Part model, mm, in its own coordinate system. A direction names the side the tool comes from. Coordinates: 2 decimals unless noted, no trailing zeros. Loops run counter-clockwise (first coordinate to the right, second up) from the corner with the lowest first, then second, coordinate; pieces in that order, holes last. Notation, with made-up numbers: M 86,5 L 105,5 A9 ccw 105,14 Z; hole C -5.5,50 d11. An arc over 180 degrees is marked long. Use a Markdown table: item, result. Add a question column.
1) Pull direction Z, two halves, no side cores. Call faces 6 (the cylindrical face through (-0.147, 1.61, 32.217)), 7 (the cylindrical face through (-30.235, 1.565, 23.183)), 8 (the flat face through (16.4, 3.175, 16.4)): released by +Z, released by -Z, zero draft, split by the parting line, or undercut.
2) Band-saw the part on D-D (z = -30). List the corners of the cut face in (x, y) (3 decimals), plus the area to 3 significant figures.
3) Pin check, flat tips, straight feed: pin 1 Ø10 at (x, y) = (-6.5, 10.5) entering from -Z; pin 2 Ø1.8 at (x, y) = (-17.78, 5.715) entering from -Z; pin 3 Ø2 at (y, z) = (5.715, -17.78) entering from +X. Stop position of each tip, or through.
4) Band-saw the part on C-C (y = 11.25). List the corners of the cut face in (x, z), plus the area to 3 significant figures.
5) Wall check: probe 1 along Y at (x, z) = (14, -28.5) (3 decimals); probe 2 along Z at (x, y) = (-16.5, 3.5); probe 3 along Z at (x, y) = (-2.5, 1.5). Give the ranges that are in metal, low to high. Write a range as from..to.
6) Band-saw the part on A-A (x = 0). List the corners of the cut face in (y, z) (3 decimals).
7) Tool access for faces 1 (the flat face through (0, 8.255, 0)), 2 (the cylindrical face through (21.804, 6.619, -6.867)), 3 (the cylindrical face through (18.9, 5.57, -10.56)), 4 (the cylindrical face through (-18.9, 5.57, 10.56)), 5 (the cylindrical face through (10.56, 5.57, 18.9)): list every direction of +Z, -Z, +X, -X, +Y, -Y with a clear straight run to the whole face (end or side of a thin tool).
8) Band-saw the part on B-B (y = 2). State how many separate pieces and enclosed holes the cut face has, plus the area to 3 significant figures.
from build123d import *

# Parameters (mm, degrees)
SKETCH2_R                 = 38.1
BOSS_EXTRUDE1_DEPTH       = 3.175
TAP_DRILL_FOR_4_40_TAP1_D = 2.2606
CIRPATTERN1_COUNT         = 8
SKETCH7_R                 = 22.86
BOSS_EXTRUDE2_DEPTH       = 6.985
SKETCH8_R                 = 19.05
CUT_EXTRUDE1_DEPTH        = 8.255
SKETCH12_W                = 1.1303
SKETCH12_H                = 38.1
CIRPATTERN2_COUNT         = 4
SKETCH14_R                = 5.08
SKETCH13_R                = 22.86


with BuildPart() as part:
    # Sketch2 → Boss-Extrude1 (new body)
    with BuildSketch(Plane(origin=(0, 0, 0), x_dir=(1, 0, 0), z_dir=(0, 1, 0))):
        Circle(SKETCH2_R)
    extrude(amount=BOSS_EXTRUDE1_DEPTH)

    # Tap Drill for #4-40 Tap1 (through all)
    with Locations(Plane(origin=(0, 0, 0), x_dir=(-1, 0, 0), z_dir=(0, -1, 0))):
        with Locations((0, -33.3375)):
            tap_drill_for_4_40_tap1 = Hole(TAP_DRILL_FOR_4_40_TAP1_D / 2)

    # CirPattern1: Tap Drill for #4-40 Tap1 ×8 about axis
    cirpattern1_axis = Axis((0, 0, 0), (0, 1, 0))
    for i in range(1, CIRPATTERN1_COUNT):
        add(tap_drill_for_4_40_tap1.rotate(cirpattern1_axis, i * 360 / CIRPATTERN1_COUNT), mode=Mode.SUBTRACT)

    # Sketch7 → Boss-Extrude2 (add)
    with BuildSketch(Plane(origin=(0, 3.175, 0), x_dir=(1, 0, 0), z_dir=(0, 1, 0))):
        Circle(SKETCH7_R)
    extrude(amount=BOSS_EXTRUDE2_DEPTH)

    # Sketch8 → Cut-Extrude1 (cut)
    with BuildSketch(Plane.XZ):
        Circle(SKETCH8_R)
    extrude(amount=-CUT_EXTRUDE1_DEPTH, mode=Mode.SUBTRACT)

    # Sketch12 → Tap Drill for #4-40 Tap2 (revolve, cut)
    with BuildSketch(Plane(origin=(-17.78, 5.715, 0), x_dir=(0, 1, 0), z_dir=(1, 0, 0))):
        with Locations((0.56515, 19.05)):
            Rectangle(SKETCH12_W, SKETCH12_H)
    tap_drill_for_4_40_tap2 = revolve(axis=Axis((-17.78, 5.715, -6.35), (0, 0, 1)), mode=Mode.SUBTRACT)

    # CirPattern2: Tap Drill for #4-40 Tap2 ×4 about axis
    cirpattern2_axis = Axis((0, 10.16, 0), (0, 1, 0))
    for i in range(1, CIRPATTERN2_COUNT):
        add(tap_drill_for_4_40_tap2.rotate(cirpattern2_axis, i * 360 / CIRPATTERN2_COUNT), mode=Mode.SUBTRACT)

    # Sketch14 → Loft2 section 0
    with BuildSketch(Plane(origin=(0, 17.78, 0), x_dir=(1, 0, 0), z_dir=(0, 1, 0))):
        Circle(SKETCH14_R)
    # Sketch13 → Loft2 section 1
    with BuildSketch(Plane(origin=(0, 10.16, 0), x_dir=(1, 0, 0), z_dir=(0, 1, 0))):
        Circle(SKETCH13_R)
    loft()


solid = part.part
Entries:
| question | item | result |
|---|---|---|
| 1 | face 6 | undercut |
| 1 | face 7 | split by the parting line |
| 1 | face 8 | zero draft |
| 2 | outline | M -23.486,0 L 23.486,0 L 23.486,3.175 L -23.486,3.175 Z |
| 2 | area | 149 mm2 |
| 3 | pin 1 | z = -22.81 |
| 3 | pin 2 | z = -15.42 |
| 3 | pin 3 | x = 15.52 |
| 4 | outline | C 0,0 d40.63 |
| 4 | area | 1,300 mm2 |
| 5 | probe 1 | 0..3.175 |
| 5 | probe 2 | -15.82..-9.52, 9.52..15.82 |
| 5 | probe 3 | -38.02..-18.89, 18.89..38.02 |
| 6 | outline | M 0,-38.1 L 3.175,-38.1 L 3.175,-34.468 L 0,-34.468 Z; M 0,-32.207 L 3.175,-32.207 L 3.175,-22.86 L 10.16,-22.86 L 17.78,-5.08 L 17.78,5.08 L 10.16,22.86 L 3.175,22.86 L 3.175,32.207 L 0,32.207 L 0,19.05 L 8.255,19.05 L 8.255,-19.05 L 0,-19.05 Z; M 0,34.468 L 3.175,34.468 L 3.175,38.1 L 0,38.1 Z |
| 7 | face 1 | -Y |
| 7 | face 2 | +Y |
| 7 | face 3 | -Z |
| 7 | face 4 | +Z |
| 7 | face 5 | +X |
| 8 | separate pieces | 1 |
| 8 | enclosed holes | 9 |
| 8 | area | 3,390 mm2 |
